Part model, mm, in its own coordinate system. A direction names the side the tool comes from. Give positions to 0.01 mm unless a question says otherwise; leave off trailing zeros. Write each loop counter-clockwise with the first axis right and the second up, starting at its lowest first coordinate (ties: lowest second). Pieces come first, ordered by that corner, then holes. Notation, with made-up numbers: (20, 29.5) - (63, 29.5) arc R13 cw to (63, 51.5) - close; hole circle Ø7 at (75.25, 34.5). An arc over 180 degrees is marked (long way). Answer as a JSON object with one key per item and string values. Group by question number.
```python
from build123d import *

# Parameters (mm, degrees)
F1_R     = 1.6
F1_W     = 5
F1_H     = 20
F2_DEPTH = 5


with BuildPart() as f2:
    # F1 (on Top) → F2 (new body)
    with BuildSketch(Plane.XY):
        Polygon((41.5, 97), (41.5, 92), (36.5, 92), (36.5, 97), (0, 97), (0, 63.5), (5, 63.5), (5, 58.5), (0, 58.5), (0, 38.5), (5, 38.5), (5, 33.5), (0, 33.5), (0, 0), (36.5, 0), (36.5, 5), (41.5, 5), (41.5, 0), (61.5, 0), (61.5, 5), (66.5, 5), (66.5, 0), (103, 0), (103, 33.5), (98, 33.5), (98, 38.5), (103, 38.5), (103, 58.5), (98, 58.5), (98, 63.5), (103, 63.5), (103, 97), (91.5, 97), (91.5, 89), (76.5, 89), (76.5, 97), (66.5, 97), (66.5, 92), (61.5, 92), (61.5, 97), align=None)
        with Locations((51.5, 2.5)):
            Circle(F1_R, mode=Mode.SUBTRACT)
        with Locations((2.5, 48.5)):
            Circle(F1_R, mode=Mode.SUBTRACT)
        with Locations((29, 48.5)):
            Rectangle(F1_W, F1_H, mode=Mode.SUBTRACT)
        with Locations((51.5, 94.5)):
            Circle(F1_R, mode=Mode.SUBTRACT)
        with Locations((74, 48.5)):
            Rectangle(F1_W, F1_H, mode=Mode.SUBTRACT)
        with Locations((100.5, 48.5)):
            Circle(F1_R, mode=Mode.SUBTRACT)
    extrude(amount=F2_DEPTH)


solid = f2.part
```
1) Mould opens along Y. For faces 5 (the flat face through (66.5, 3, 2)), 6 (the flat face through (72, 97, 2)), 7 (the flat face through (100, 38.5, 2)) say: pulls with the +Y half, pulls with the -Y half, needs draft (parallel to the pull), parting line crosses it, or undercut.
2) Drop flat-ended pins along their axis: P1, Ø2.5, axis at y = 36.5, z = 3.5, coming from the +X side; P2, Ø2.5, axis at x = 84.5, z = 3, coming from the +Y side; P3, Ø2.5, axis at x = 51.5, y = 2.5, coming from the -Z side. Give the stop position or say it passes through.
3) Band-saw the part on C-C (y = 2.5). List the corners of the cut face in (x, z).
4) Band-saw the part on D-D (x = 51.5). List the corners of the cut face in (y, z), plus the area to 3 significant figures.
5) Probe line 1 (Y direction, x = 51.5, z = 3.65); line 2 (X direction, y = 94.5, z = 2.55); line 3 (X direction, y = 50.5, z = 0.8). List the from-to ranges inside material, lowest first.
6) Band-saw the part on A-A (y = 94.5). List the corners of the cut face in (x, z), plus the area to 3 significant figures.
7) Which spindle directions (+Z, -Z, +X, -X, +Y, -Y) get a long thin tool onto all of the face, cutting with end or side? Do faces 1 (the flat face through (2, 63.5, 2)), 2 (the flat face through (61.5, 94, 2)), 3 (the flat face through (98, 36, 2)), 4 (the flat face through (29, 38.5, 2)). Say none if no direction does.
8) Band-saw the part on B-B (x = 100.5). List the corners of the cut face in (y, z).
Verdict:
{
 "1": {"face 5": "needs draft", "face 6": "pulls with the +Y half", "face 7": "undercut"},
 "2": {"P1": "x = 98", "P2": "y = 89", "P3": "through"},
 "3": {"outline": "(0, 0) - (36.5, 0) - (36.5, 5) - (0, 5) - close; (41.5, 0) - (49.9, 0) - (49.9, 5) - (41.5, 5) - close; (53.1, 0) - (61.5, 0) - (61.5, 5) - (53.1, 5) - close; (66.5, 0) - (103, 0) - (103, 5) - (66.5, 5) - close"},
 "4": {"outline": "(0, 0) - (0.9, 0) - (0.9, 5) - (0, 5) - close; (4.1, 0) - (92.9, 0) - (92.9, 5) - (4.1, 5) - close; (96.1, 0) - (97, 0) - (97, 5) - (96.1, 5) - close", "area": "453 mm2"},
 "5": {"line 1": "0 to 0.9, 4.1 to 92.9, 96.1 to 97", "line 2": "0 to 36.5, 41.5 to 49.9, 53.1 to 61.5, 66.5 to 76.5, 91.5 to 103", "line 3": "0 to 26.5, 31.5 to 71.5, 76.5 to 103"},
 "6": {"outline": "(0, 0) - (36.5, 0) - (36.5, 5) - (0, 5) - close; (41.5, 0) - (49.9, 0) - (49.9, 5) - (41.5, 5) - close; (53.1, 0) - (61.5, 0) - (61.5, 5) - (53.1, 5) - close; (66.5, 0) - (76.5, 0) - (76.5, 5) - (66.5, 5) - close; (91.5, 0) - (103, 0) - (103, 5) - (91.5, 5) - close", "area": "374 mm2"},
 "7": {"face 1": "+Z, -Z, -X", "face 2": "+Z, -Z, +Y", "face 3": "+Z, -Z, +X", "face 4": "+Z, -Z"},
 "8": {"outline": "(0, 0) - (33.5, 0) - (33.5, 5) - (0, 5) - close; (38.5, 0) - (46.9, 0) - (46.9, 5) - (38.5, 5) - close; (50.1, 0) - (58.5, 0) - (58.5, 5) - (50.1, 5) - close; (63.5, 0) - (97, 0) - (97, 5) - (63.5, 5) - close"}
}
